Geometry check sheet. Reference: the model listing, model coordinates, mm. Round coordinates to 2 decimals unless told otherwise and drop trailing zeros. Write each loop counter-clockwise with the first axis right and the second up, starting at its lowest first coordinate (ties: lowest second). Pieces come first, ordered by that corner, then holes. Notation, with made-up numbers: M 60,-40 L 76,-40 A8 cw 76,-32 Z; hole C 26,10.25 d8. An arc over 180 degrees is marked long. Answer in a Markdown table with one row per item. Add a question column.
from build123d import *

# Parameters (mm, degrees)
ESQUISSE1_W             = 75
ESQUISSE1_H             = 20
BOSS_EXTRU_1_DEPTH      = 5
ESQUISSE2_W             = 5
ESQUISSE2_H             = 5
BOSS_EXTRU_2_DEPTH      = 5
ESQUISSE3_R             = 1.5
ENL_V_MAT_EXTRU_1_DEPTH = 79.262379212
ESQUISSE4_R             = 1.5
ENL_V_MAT_EXTRU_2_DEPTH = 79.262379212
ESQUISSE5_R             = 3
ENL_V_MAT_EXTRU_3_DEPTH = 3


with BuildPart() as part:
    # Esquisse1 → Boss.-Extru.1 (new body)
    with BuildSketch(Plane.XY):
        with Locations((37.5, 10)):
            Rectangle(ESQUISSE1_W, ESQUISSE1_H)
    extrude(amount=BOSS_EXTRU_1_DEPTH)

    # Esquisse2 → Boss.-Extru.2 (add)
    with BuildSketch(Plane.XY.offset(5)):
        with Locations((70.5, 17.5)):
            Rectangle(ESQUISSE2_W, ESQUISSE2_H)
        with Locations((70.5, 2.5)):
            Rectangle(ESQUISSE2_W, ESQUISSE2_H)
    extrude(amount=BOSS_EXTRU_2_DEPTH)

    # Esquisse3 → Enlèv. mat.-Extru.1 (cut, through all)
    with BuildSketch(Plane.XZ):
        with Locations(Location((70.5, 7.5, 0), (0, 0, 270))):
            Circle(ESQUISSE3_R)
        with BuildLine():
            Line((68, 10), (68, 7.5))
            ThreePointArc((68, 7.5), (68.732233047, 9.267766953), (70.5, 10))
            Line((70.5, 10), (68, 10))
        make_face()
        with BuildLine():
            Line((73, 10), (70.5, 10))
            ThreePointArc((70.5, 10), (72.267766953, 9.267766953), (73, 7.5))
            Line((73, 7.5), (73, 10))
        make_face()
    extrude(amount=-ENL_V_MAT_EXTRU_1_DEPTH, mode=Mode.SUBTRACT)

    # Esquisse4 → Enlèv. mat.-Extru.2 (cut, through all)
    with BuildSketch(Plane(origin=(0, 0, 0), x_dir=(-1, 0, 0), z_dir=(0, 0, -1))):
        with Locations((-5, 6.666666667)):
            Circle(ESQUISSE4_R)
        with Locations((-5, 13.333333333)):
            Circle(ESQUISSE4_R)
    extrude(amount=-ENL_V_MAT_EXTRU_2_DEPTH, mode=Mode.SUBTRACT)

    # Esquisse5 → Enlèv. mat.-Extru.3 (cut)
    with BuildSketch(Plane(origin=(0, 0, 0), x_dir=(-1, 0, 0), z_dir=(0, 0, -1))):
        with Locations((-5, 6.666666667)):
            Circle(ESQUISSE5_R)
        with Locations((-5, 13.333333333)):
            Circle(ESQUISSE5_R)
    extrude(amount=-ENL_V_MAT_EXTRU_3_DEPTH, mode=Mode.SUBTRACT)


solid = part.part
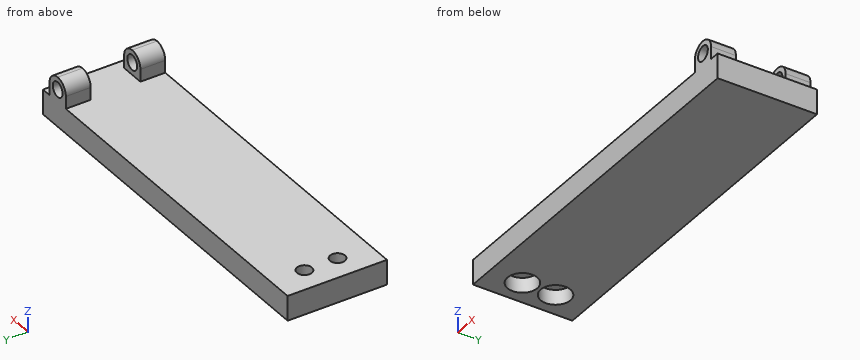
Item 1: Gauge pin test, flat ends, axial feed: pin 1 Ø4 at (x, y) = (5, 6.67) entering from -Z; pin 2 Ø3 at (y, z) = (17, 7) entering from +X; pin 3 Ø0.8 at (y, z) = (2, 6.5) entering from -X. Record the tip position at first contact, or that the pin passes through.
Item 2: Section check A-A, the plane x = 5. Record the boundary of the cut face in (y, z), and give its area (3 significant figures).
Item 3: Section check B-B, the plane y = 2.25. Record the boundary of the cut face in (x, z).
Item 4: Section check C-C, the plane z = 8.25. Record the boundary of the cut face in (x, y).
Item 5: Section check D-D, the plane x = 41.5. Record the boundary of the cut face in (y, z), and give its area (3 significant figures).
Item 6: Scan lines: probe 1 along Y at (x, z) = (5, 3.6); probe 2 along X at (y, z) = (18.35, 7.5); probe 3 along Y at (x, z) = (69.5, 9.25). Record each from-to range of solid material in increasing order. Write a range as from..to.
Result sheet:
| question | item | result |
|---|---|---|
| 1 | pin 1 | stops at z = 3 |
| 1 | pin 2 | stops at x = 73 |
| 1 | pin 3 | stops at x = 68 |
| 2 | outline | M 0,0 L 3.67,0 L 3.67,3 L 5.17,3 L 5.17,5 L 0,5 Z; M 8.17,3 L 9.67,3 L 9.67,0 L 10.33,0 L 10.33,3 L 11.83,3 L 11.83,5 L 8.17,5 Z; M 14.83,3 L 16.33,3 L 16.33,0 L 20,0 L 20,5 L 14.83,5 Z |
| 2 | area | 52.0 mm^2 |
| 3 | outline | M 0,0 L 75,0 L 75,5 L 73,5 L 73,7.5 A2.5 ccw 68,7.5 L 68,5 L 0,5 Z; hole C 70.5,7.5 d3 |
| 4 | outline | M 68.12,0 L 69.2,0 L 69.2,5 L 68.12,5 Z; M 68.12,15 L 69.2,15 L 69.2,20 L 68.12,20 Z; M 71.8,0 L 72.88,0 L 72.88,5 L 71.8,5 Z; M 71.8,15 L 72.88,15 L 72.88,20 L 71.8,20 Z |
| 5 | outline | M 0,0 L 20,0 L 20,5 L 0,5 Z |
| 5 | area | 100 mm^2 |
| 6 | probe 1 | y = 0..5.17, 8.17..11.83, 14.83..20 |
| 6 | probe 2 | x = 68..69, 72..73 |
| 6 | probe 3 | y = 0..5, 15..20 |
